Work out the finished part from the listing and answer in its coordinate system (mm). Coordinates: 2 decimals unless noted, no trailing zeros. Order: outer loops, then holes, each group sorted by start corner. A loop starts at its lowest first (then second) coordinate and runs counter-clockwise, first axis right, second up.
```python
from build123d import *

# Parameters (mm, degrees)
SKETCH2_R          = 2
CUT_EXTRUDE1_DEPTH = 20
CIRPATTERN1_COUNT  = 10


with BuildPart() as part:
    # Sketch1 → Revolve2 (revolve)
    with BuildSketch(Plane.XY, mode=Mode.PRIVATE) as revolve2_sk:
        Polygon((-65, 60), (-70, 60), (-176.700455888, 0), (-160, 0), (-80, 45), (-80, 40), (0, 40), (0, 50), (-70, 50), (-70, 55), (-65, 55), align=None)
    revolve(revolve2_sk.sketch.rotate(Axis((-123.889506721, 0, 0), (1, 0, 0)), 180), axis=Axis((-123.889506721, 0, 0), (1, 0, 0)))

    # Sketch2 → Cut-Extrude1 (cut)
    with BuildSketch(Plane(origin=(0, 0, 0), x_dir=(0, 0, -1), z_dir=(1, 0, 0))):
        with Locations(Location((0, 45, 0), (0, 0, 90))):
            Circle(SKETCH2_R)
    cut_extrude1 = extrude(amount=-CUT_EXTRUDE1_DEPTH, mode=Mode.SUBTRACT)

    # CirPattern1: Cut-Extrude1 ×10 about axis
    cirpattern1_axis = Axis((0, 0, 0), (1, 0, 0))
    for i in range(1, CIRPATTERN1_COUNT):
        add(cut_extrude1.rotate(cirpattern1_axis, i * 360 / CIRPATTERN1_COUNT), mode=Mode.SUBTRACT)


solid = part.part
```
1. The mould has two halves that part along Z. Classify faces 1 (the flat face through (-80, 30.2, 26.5)), 2 (the flat face through (-20, 45, 0)), 3 (the flat face through (0, -34, 22)): released by +Z, released by -Z, zero draft, split by the parting line, or undercut.
2. Flat-ended cylindrical pins translate along their axes: pin 1 (4 mm diameter, centred on x = -127, y = 12.5, fed in from +Z); pin 2 (4 mm diameter, centred on x = -42.5, z = 14.5, fed in from -Y); pin 3 (5 mm diameter, centred on y = 36.41, z = -26.45, fed in from +X); pin 4 (3 mm diameter, centred on y = 13.91, z = -42.8, fed in from +X). Find the tip coordinate at first contact, or state that the pin passes through.
3. Consider probe 1 along Z at (x, y) = (-38.5, -1); probe 2 along Z at (x, y) = (-14.5, 2.5); probe 3 along Y at (x, z) = (-13, -35.5). Determine where each line is inside the solid, lowest interval first.
4. The part is cut by section B-B (x = -88.5). Determine the outline of the cut face in (y, z), plus the area to 3 significant figures.
5. The part is cut by section A-A (x = -54.5). Determine the outline of the cut face in (y, z), plus the area to 3 significant figures.
Worked out:
1. face 1: undercut
1. face 2: undercut
1. face 3: zero draft
2. pin 1: stops at z = 26.54
2. pin 2: stops at y = -48.41
2. pin 3: stops at x = 0
2. pin 4: stops at x = -20
3. probe 1: z = -49.99 to -39.99, 39.99 to 49.99
3. probe 2: z = -49.94 to -39.92, 39.92 to 49.94
3. probe 3: y = -35.21 to -18.43, 18.43 to 35.21
4. outline: circle Ø99.19 at (0, 0); hole circle Ø80.44 at (0, 0)
4. area: 2,650 mm2
5. outline: circle Ø100 at (0, 0); hole circle Ø80 at (0, 0)
5. area: 2,830 mm2
